Input: part model. Units: mm. Frame: model coordinates. A direction names the side the tool comes from. Give positions to 0.01 mm unless a question says otherwise; leave off trailing zeros. Order: outer loops, then holes, each group sorted by start corner. A loop starts at its lowest first (then second) coordinate and runs counter-clockwise, first axis right, second up. Notation, with made-up numbers: (5, 36) - (40, 36) arc R19 cw to (40, 71) - close; hole circle Ø9 at (78.25, 57). An arc over 180 degrees is marked (long way). Answer in a Markdown table with one row per item. Add a question column.
from build123d import *

# Parameters (mm, degrees)
SKETCH_W        = 14
SKETCH_H        = 24
PAD_DEPTH       = 5
SKETCH003_R     = 1
POCKET_DEPTH    = 5
SKETCH004_R     = 1
POCKET001_DEPTH = 6


with BuildPart() as part:
    # Sketch → Pad (new body, symmetric)
    with BuildSketch(Plane.XZ):
        Polygon((-30, 0), (30, 0), (30, 2), (24, 2), (24, 102), (-24, 102), (-24, 2), (-30, 2), align=None)
        with Locations((0, 82)):
            Rectangle(SKETCH_W, SKETCH_H, mode=Mode.SUBTRACT)
    extrude(amount=PAD_DEPTH, both=True)

    # Sketch003 → Pocket (cut)
    with BuildSketch(Plane.XY):
        with Locations((-27, 0)):
            Circle(SKETCH003_R)
        with Locations((27, 0)):
            Circle(SKETCH003_R)
    extrude(amount=POCKET_DEPTH, mode=Mode.SUBTRACT)

    # Sketch004 → Pocket001 (cut)
    with BuildSketch(Plane.XZ):
        with Locations((0, 67.5)):
            Circle(SKETCH004_R)
        with Locations((0, 95.5)):
            Circle(SKETCH004_R)
    extrude(amount=-POCKET001_DEPTH, mode=Mode.SUBTRACT)


solid = part.part
Q1. Section A-A, the plane x = -27. Return loops of the section in (y, z), then the cut area to 3 significant figures.
Q2. Section D-D, the plane z = 95.5. Return loops of the section in (x, y).
Q3. Contact query for flat-ended pins moving along their axis: P1, Ø3, axis at y = -1, z = 87.5, coming from the +X side; P2, Ø1.2, axis at x = 0, z = 67.5, coming from the +Y side; P3, Ø2.5, axis at x = 27, y = 0, coming from the +Z side; P4, Ø2, axis at x = 0, z = 68, coming from the +Y side. Output: stop coordinate, or through.
Q4. Pull-direction query (Y, two-part tool) for faces 4 (the cylindrical face through (26, 0, 1)), 5 (the flat face through (0, -5, 52)), 6 (the cylindrical face through (0.46, 2.46, 94.61)); classes: +Y half, -Y half, draft (parallel to the pull), parting line (faces both ways), or undercut.
Q5. Section B-B, the plane y = -2. Return loops of the section in (x, z).
Q6. Section C-C, the plane z = 80.5. Return loops of the section in (x, y), then the cut area to 3 significant figures.
Q7. Line query: probe 1 along Z at (x, y) = (0, 2.15); probe 2 along X at (y, z) = (0, 0.65); probe 3 along X at (y, z) = (2.7, 67.5). Output: solid intervals per line, ascending.
Q8. Access query for faces 1 (the flat face through (-27, -1.2, 2)), 2 (the flat face through (7, 0, 82)), 3 (the flat face through (0, 0, 68)). Directions: +Z, -Z, +X, -X, +Y, -Y. A direction counts if a zero-diameter tool reaches every point of the face in a straight line with its end or side. Return the directions, or none.
Computed:
| question | item | result |
|---|---|---|
| 1 | outline | (-5, 0) - (-1, 0) - (-1, 2) - (-5, 2) - close; (1, 0) - (5, 0) - (5, 2) - (1, 2) - close |
| 1 | area | 16.0 mm^2 |
| 2 | outline | (-24, -5) - (24, -5) - (24, 5) - (1, 5) - (1, 0) - (-1, 0) - (-1, 5) - (-24, 5) - close |
| 3 | P1 | stops at x = 24 |
| 3 | P2 | stops at y = 0 |
| 3 | P3 | stops at z = 2 |
| 3 | P4 | stops at y = 5 |
| 4 | face 4 | undercut |
| 4 | face 5 | -Y half |
| 4 | face 6 | draft |
| 5 | outline | (-30, 0) - (30, 0) - (30, 2) - (24, 2) - (24, 102) - (-24, 102) - (-24, 2) - (-30, 2) - close; hole (-7, 70) - (7, 70) - (7, 94) - (-7, 94) - close |
| 6 | outline | (-24, -5) - (-7, -5) - (-7, 5) - (-24, 5) - close; (7, -5) - (24, -5) - (24, 5) - (7, 5) - close |
| 6 | area | 340 mm^2 |
| 7 | probe 1 | z = 0 to 66.5, 68.5 to 70, 94 to 94.5, 96.5 to 102 |
| 7 | probe 2 | x = -30 to -28, -26 to 26, 28 to 30 |
| 7 | probe 3 | x = -24 to -1, 1 to 24 |
| 8 | face 1 | +Z, -X, +Y, -Y |
| 8 | face 2 | +Y, -Y |
| 8 | face 3 | +Y |
